```python
from build123d import *

# Parameters (mm, degrees)
SKETCH1_R             = 5
BOSS_EXTRUDE1_DEPTH   = 10
BOSS_EXTRUDE1_2_DEPTH = 10
BOSS_EXTRUDE1_3_DEPTH = 10
BOSS_EXTRUDE1_4_DEPTH = 10
BOSS_EXTRUDE1_5_DEPTH = 10
BOSS_EXTRUDE1_6_DEPTH = 10
SKETCH2_R             = 30
SKETCH2_R_2           = 4.05
SKETCH2_R_3           = 2
BOSS_EXTRUDE2_DEPTH   = 10
CUT_EXTRUDE1_DEPTH    = 5.5


with BuildPart() as part:
    # Sketch1 → Boss-Extrude1 (new body)
    with BuildSketch(Plane.XY):
        with Locations((20, 0)):
            Circle(SKETCH1_R)
    extrude(amount=BOSS_EXTRUDE1_DEPTH)



with BuildPart() as body_2:
    # Sketch1 → Boss-Extrude1 2 (new body)
    with BuildSketch(Plane.XY):
        with Locations((10, -17.320508076)):
            Circle(SKETCH1_R)
    extrude(amount=BOSS_EXTRUDE1_2_DEPTH)


with BuildPart() as body_3:
    # Sketch1 → Boss-Extrude1 3 (new body)
    with BuildSketch(Plane.XY):
        with Locations((-10, -17.320508076)):
            Circle(SKETCH1_R)
    extrude(amount=BOSS_EXTRUDE1_3_DEPTH)


with BuildPart() as body_4:
    # Sketch1 → Boss-Extrude1 4 (new body)
    with BuildSketch(Plane.XY):
        with Locations((-20, 0)):
            Circle(SKETCH1_R)
    extrude(amount=BOSS_EXTRUDE1_4_DEPTH)


with BuildPart() as body_5:
    # Sketch1 → Boss-Extrude1 5 (new body)
    with BuildSketch(Plane.XY):
        with Locations((-10, 17.320508076)):
            Circle(SKETCH1_R)
    extrude(amount=BOSS_EXTRUDE1_5_DEPTH)


with BuildPart() as body_6:
    # Sketch1 → Boss-Extrude1 6 (new body)
    with BuildSketch(Plane.XY):
        with Locations((10, 17.320508076)):
            Circle(SKETCH1_R)
    extrude(amount=BOSS_EXTRUDE1_6_DEPTH)


with BuildPart() as part_1:
    add(part.part)

    add(body_2.part)  # Boss-Extrude2 merges body 2

    add(body_3.part)  # Boss-Extrude2 merges body 3

    add(body_4.part)  # Boss-Extrude2 merges body 4

    add(body_5.part)  # Boss-Extrude2 merges body 5

    add(body_6.part)  # Boss-Extrude2 merges body 6
    # Sketch2 → Boss-Extrude2 (add)
    with BuildSketch(Plane.XY.offset(10)):
        Circle(SKETCH2_R)
        Circle(SKETCH2_R_2, mode=Mode.SUBTRACT)
        with Locations((-0.00055318, 12.499999988)):
            Circle(SKETCH2_R_3, mode=Mode.SUBTRACT)
        with Locations((10.825540946, 6.251345088)):
            Circle(SKETCH2_R_3, mode=Mode.SUBTRACT)
        with Locations((10.827094127, -6.2486549)):
            Circle(SKETCH2_R_3, mode=Mode.SUBTRACT)
        with Locations((0.00255318, -12.499999988)):
            Circle(SKETCH2_R_3, mode=Mode.SUBTRACT)
        with Locations((-10.823540946, -6.251345088)):
            Circle(SKETCH2_R_3, mode=Mode.SUBTRACT)
        with Locations((-10.825094127, 6.2486549)):
            Circle(SKETCH2_R_3, mode=Mode.SUBTRACT)
    extrude(amount=BOSS_EXTRUDE2_DEPTH)

    # Sketch5 → Cut-Extrude1 (cut)
    with BuildSketch(Plane(origin=(0, 0, 10), x_dir=(-1, 0, 0), z_dir=(0, 0, -1))):
        Polygon((7.621014042, 0.012040338), (3.800079783, 6.606011932), (-3.82093426, 6.593971594), (-7.621014042, -0.012040338), (-3.800079783, -6.606011932), (3.82093426, -6.593971594), align=None)
    extrude(amount=-CUT_EXTRUDE1_DEPTH, mode=Mode.SUBTRACT)


solid = part_1.part
```
Source: CAD feature listing. Evaluate the final solid. Frame: model axes, mm. A direction names the side the tool comes from. Round coordinates to 2 decimals unless told otherwise and drop trailing zeros. Loops run counter-clockwise (first coordinate to the right, second up) from the corner with the lowest first, then second, coordinate; pieces in that order, holes last. Notation, with made-up numbers: M 20,38.5 L 72,38.5 A12 cw 72,42.5 Z; hole C 11,1 d5. An arc over 180 degrees is marked long. Use a Markdown table: item, result. Add a question column.
1. Section query A-A on x = 0. Return the cut outline in (y, z).
2. Section query D-D on y = -16.5. Return the cut outline in (x, z).
3. Section query C-C on x = 19.5. Return the cut outline in (y, z), then the cut area to 3 significant figures.
4. Contact query for flat-ended pins moving along their axis: P1, Ø2.5, axis at x = 0, y = 12.5, coming from the +Z side; P2, Ø4.5, axis at x = 10.83, y = -6.25, coming from the -Z side; P3, Ø8, axis at x = 20.5, z = 13.5, coming from the +Y side; P4, Ø4, axis at y = -18, z = 12.5, coming from the +X side. Output: stop coordinate, or through.
5. Mould query, pull axis Y, two halves, no side actions, for faces 1 (the flat face through (20, 0, 0)), 2 (the cylindrical face through (14.77, -15.82, 4.93)), 3 (the cylindrical face through (-29.97, 1.32, 14.93)). Classes: pulls with the +Y half, pulls with the -Y half, needs draft (parallel to the pull), parting line crosses it, or undercut.
6. Reachability of faces 4 (the cylindrical face through (0.93, -14.27, 14.93)), 5 (the flat face through (-5.74, 3.26, 12.71)) from +Z, -Z, +X, -X, +Y, -Y: full face, straight path, thin tool, end or side. Return the list, or none.
7. Line query: line 1 (Z direction, x = 20.5, y = -17); line 2 (Z direction, x = 0, y = -5.5); line 3 (Y direction, x = 5.5, z = 5.75). Output: solid intervals per line, ascending.
8. Section query B-B on z = 12. Return the cut outline in (x, y).
Reported:
| question | item | result |
|---|---|---|
| 1 | outline | M -30,10 L -14.5,10 L -14.5,20 L -30,20 Z; M -10.5,10 L -6.6,10 L -6.6,15.5 L -4.05,15.5 L -4.05,20 L -10.5,20 Z; M 4.05,15.5 L 6.6,15.5 L 6.6,10 L 10.5,10 L 10.5,20 L 4.05,20 Z; M 14.5,10 L 30,10 L 30,20 L 14.5,20 Z |
| 2 | outline | M -25.05,10 L -14.93,10 L -14.93,0 L -5.07,0 L -5.07,10 L 5.07,10 L 5.07,0 L 14.93,0 L 14.93,10 L 25.05,10 L 25.05,20 L -25.05,20 Z |
| 3 | outline | M -22.8,10 L -4.97,10 L -4.97,0 L 4.97,0 L 4.97,10 L 22.8,10 L 22.8,20 L -22.8,20 Z |
| 3 | area | 555 mm² |
| 4 | P1 | passes through |
| 4 | P2 | stops at z = 10 |
| 4 | P3 | stops at y = 25.05 |
| 4 | P4 | stops at x = 25.38 |
| 5 | face 1 | needs draft |
| 5 | face 2 | undercut |
| 5 | face 3 | parting line crosses it |
| 6 | face 4 | +Z, -Z |
| 6 | face 5 | -Z |
| 7 | line 1 | z = 10 to 20 |
| 7 | line 2 | z = 15.5 to 20 |
| 7 | line 3 | y = -19.5 to -15.14, 15.14 to 19.5 |
| 8 | outline | C 0,0 d60; hole C -10.83,6.25 d4; hole C -10.82,-6.25 d4; hole M -7.62,0.01 L -3.82,-6.59 L 3.8,-6.61 L 7.62,-0.01 L 3.82,6.59 L -3.8,6.61 Z; hole C 0,-12.5 d4; hole C 0,12.5 d4; hole C 10.83,-6.25 d4; hole C 10.83,6.25 d4 |
